Verification items for the finished model (mm, model axes). Coordinates: 2 decimals unless noted, no trailing zeros. Loops run counter-clockwise (first coordinate to the right, second up) from the corner with the lowest first, then second, coordinate; pieces in that order, holes last. Notation, with made-up numbers: (24, 24) -> (82, 24) arc R8 ccw to (82, 34) -> close; hole circle Ø4 at (6.5, -10). An arc over 180 degrees is marked (long way). Answer as a JSON object with one key per item and string values. Group by question number.
Q1. Scan lines: L1, parallel to Y at x = 105.5, z = 2.2; L2, parallel to Y at x = 111.5, z = 2.75; L3, parallel to Y at x = 64.5, z = 1.6. Record each from-to range of solid material in increasing order.
Q2. Cross-section at A-A on x = 49. Record the boundary of the cut face in (y, z) (3 decimals).
Q3. Cross-section at B-B on x = -95.25. Record the boundary of the cut face in (y, z) (3 decimals).
Q4. Cross-section at C-C on z = 0.6. Give the number of separate pieces and of enclosed holes in the cut face, and give its area (3 significant figures).
Q5. Release check for a two-part mould opening along Y. For faces 1 (the flat face through (-3, 2, 3.175)), 2 (the cylindrical face through (-137.63, -46.04, 1.61)) record: released by +Y, released by -Y, zero draft, split by the parting line, or undercut.
Q6. Gauge pin test, flat ends, axial feed: pin 1 Ø3 at (x, y) = (145.5, -132.4) entering from +Z; pin 2 Ø8 at (x, y) = (76.5, -100.5) entering from -Z. Record the tip position at first contact, or that the pin passes through.
```python
from build123d import *

# Parameters (mm, degrees)
SKETCH1_W           = 457.2
SKETCH1_H           = 304.8
ACRYLIC_PANEL_DEPTH = 3.175
SKETCH2_R           = 2.6
SKETCH2_R_2         = 57.5
SKETCH2_R_3         = 1.85
SKETCH2_R_4         = 1.7
SKETCH2_W           = 3.175
SKETCH2_H           = 15
SKETCH2_W_2         = 19.5
SKETCH2_H_2         = 12
SKETCH2_W_3         = 27.5
SKETCH2_H_3         = 47
CUT_EXTRUDE1_DEPTH  = 275.761352131


with BuildPart() as part:
    # Sketch1 → Acrylic Panel (new body)
    with BuildSketch(Plane.XY):
        Rectangle(SKETCH1_W, SKETCH1_H)
    extrude(amount=ACRYLIC_PANEL_DEPTH)

    # Sketch2 → Cut-Extrude1 (cut, through all)
    with BuildSketch(Plane.XY.offset(3.175)):
        with Locations((-147.75, -32.4)):
            Circle(SKETCH2_R)
        with Locations((-42.75, -32.4)):
            Circle(SKETCH2_R)
        with Locations((-147.75, -137.4)):
            Circle(SKETCH2_R)
        with Locations((-42.75, -137.4)):
            Circle(SKETCH2_R)
        with Locations((-95.25, -84.9)):
            Circle(SKETCH2_R_2)
        with Locations((25, -92.4)):
            Circle(SKETCH2_R_3)
        with Locations((64.5, -92.4)):
            Circle(SKETCH2_R_3)
        with Locations((105.5, -132.4)):
            Circle(SKETCH2_R_4)
        with Locations((130.5, -132.4)):
            Circle(SKETCH2_R_4)
        with Locations((145.5, -132.4)):
            Circle(SKETCH2_R_4)
        with Locations((170.5, -132.4)):
            Circle(SKETCH2_R_4)
        with Locations((145.5, -112.4)):
            Circle(SKETCH2_R_4)
        with Locations((170.5, -112.4)):
            Circle(SKETCH2_R_4)
        with Locations((145.5, -92.4)):
            Circle(SKETCH2_R_4)
        with Locations((170.5, -92.4)):
            Circle(SKETCH2_R_4)
        with Locations((105.5, -112.4)):
            Circle(SKETCH2_R_4)
        with Locations((130.5, -112.4)):
            Circle(SKETCH2_R_4)
        with Locations((105.5, -92.4)):
            Circle(SKETCH2_R_4)
        with Locations((130.5, -92.4)):
            Circle(SKETCH2_R_4)
        with Locations((0, -50.8)):
            Rectangle(SKETCH2_W, SKETCH2_H)
        with Locations((190.5, -50.8)):
            Rectangle(SKETCH2_W, SKETCH2_H)
        with Locations((-190.5, -50.8)):
            Rectangle(SKETCH2_W, SKETCH2_H)
        with Locations((118, -132.4)):
            Rectangle(SKETCH2_W_2, SKETCH2_H_2)
        with Locations((158, -132.4)):
            Rectangle(SKETCH2_W_2, SKETCH2_H_2)
        with Locations((158, -112.4)):
            Rectangle(SKETCH2_W_2, SKETCH2_H_2)
        with Locations((158, -92.4)):
            Rectangle(SKETCH2_W_2, SKETCH2_H_2)
        with Locations((118, -112.4)):
            Rectangle(SKETCH2_W_2, SKETCH2_H_2)
        with Locations((118, -92.4)):
            Rectangle(SKETCH2_W_2, SKETCH2_H_2)
        with Locations((44.75, -92.4)):
            Rectangle(SKETCH2_W_3, SKETCH2_H_3)
    extrude(amount=-CUT_EXTRUDE1_DEPTH, mode=Mode.SUBTRACT)


solid = part.part
```
Computed values:
{
 "1": {"L1": "y = -152.4 to -134.1, -130.7 to -114.1, -110.7 to -94.1, -90.7 to 152.4", "L2": "y = -152.4 to -138.4, -126.4 to -118.4, -106.4 to -98.4, -86.4 to 152.4", "L3": "y = -152.4 to -94.25, -90.55 to 152.4"},
 "2": {"outline": "(-152.4, 0) -> (-115.9, 0) -> (-115.9, 3.175) -> (-152.4, 3.175) -> close; (-68.9, 0) -> (152.4, 0) -> (152.4, 3.175) -> (-68.9, 3.175) -> close"},
 "3": {"outline": "(-152.4, 0) -> (-142.4, 0) -> (-142.4, 3.175) -> (-152.4, 3.175) -> close; (-27.4, 0) -> (152.4, 0) -> (152.4, 3.175) -> (-27.4, 3.175) -> close"},
 "4": {"separate pieces": "1", "enclosed holes": "29", "area": "126,000 mm²"},
 "5": {"face 1": "zero draft", "face 2": "undercut"},
 "6": {"pin 1": "passes through", "pin 2": "stops at z = 0"}
}
